Part model, mm, in its own coordinate system. Face numbers are marked on the shaded views. A direction names the side the tool comes from. Round coordinates to 2 decimals unless told otherwise and drop trailing zeros. Order: outer loops, then holes, each group sorted by start corner. A loop starts at its lowest first (then second) coordinate and runs counter-clockwise, first axis right, second up. Notation, with made-up numbers: (6, 9.5) - (32, 9.5) arc R12 cw to (32, 24.5) - close; hole circle Ø4 at (-13, 63.5). An arc over 180 degrees is marked (long way). Return JSON: item names as keys, results as strings. Group by question number.
Item 1: Saw through at A-A on y = -28. List the corners of the cut face in (x, z).
Item 2: Drop flat-ended pins along their axis: pin 1 (3 mm diameter, centred on y = -13, z = 0.5, fed in from -X); pin 2 (5 mm diameter, centred on y = 3.5, z = 3, fed in from +X); pin 3 (3 mm diameter, centred on y = -27.5, z = 2, fed in from +X). Give the stop position or say it passes through.
Item 3: Probe probe 1 along X at (y, z) = (26.25, 0); probe 2 along Z at (x, y) = (-25, 23.5); probe 3 along Y at (x, z) = (-17, -4.5). List the from-to ranges inside material, lowest first.
Item 4: Saw through at D-D on z = 3.5. List the corners of the cut face in (x, y).
Item 5: Two-plate mould, pull along Y, no slides. Class the marked faces 1, 2, 3 and 4: released by +Y, released by -Y, zero draft, split by the parting line, or undercut.
Item 6: Tool access for the marked faces 5 and 6: list every direction of +Z, -Z, +X, -X, +Y, -Y with a clear straight run to the whole face (end or side of a thin tool).
Item 7: Saw through at C-C on y = -13.5. List the corners of the cut face in (x, z).
Item 8: Saw through at B-B on z = 0. State how many separate pieces and enclosed holes the cut face has, and give its area (3 significant figures).
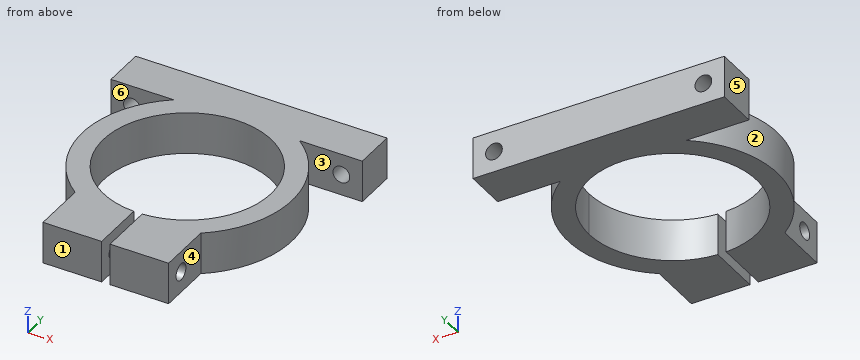
```python
from build123d import *

# Parameters (mm, degrees)
CYLINDER002_R     = 2
CYLINDER002_DEPTH = 10
CYLINDER001_R     = 20
CYLINDER001_DEPTH = 10
CYLINDER004_R     = 2
CYLINDER004_DEPTH = 30
BOX002_W          = 2
BOX002_H          = 15
BOX002_DEPTH      = 10
CYLINDER003_R     = 2
CYLINDER003_DEPTH = 10
BOX_W             = 60
BOX_H             = 10
BOX_DEPTH         = 10
BOX001_W          = 30
BOX001_H          = 15
BOX001_DEPTH      = 10
CYLINDER_R        = 25
CYLINDER_DEPTH    = 10


with BuildPart() as cylinder002:
    # Cylinder002 → Cylinder002 (new body)
    with BuildSketch(Plane(origin=(25, 20, 0), x_dir=(1, 0, 0), z_dir=(0, 1, 0))):
        Circle(CYLINDER002_R)
    extrude(amount=CYLINDER002_DEPTH)


with BuildPart() as cylinder001:
    # Cylinder001 → Cylinder001 (new body)
    with BuildSketch(Plane.XY.offset(-5)):
        Circle(CYLINDER001_R)
    extrude(amount=CYLINDER001_DEPTH)


with BuildPart() as cylinder004:
    # Cylinder004 → Cylinder004 (new body)
    with BuildSketch(Plane(origin=(-15, -28, 0), x_dir=(0, 0, -1), z_dir=(1, 0, 0))):
        Circle(CYLINDER004_R)
    extrude(amount=CYLINDER004_DEPTH)


with BuildPart() as cube002:
    # Box002 → Box002 (new body)
    with BuildSketch(Plane(origin=(-1, -33, -5), x_dir=(1, 0, 0), z_dir=(0, 0, 1))):
        with Locations((1, 7.5)):
            Rectangle(BOX002_W, BOX002_H)
    extrude(amount=BOX002_DEPTH)


with BuildPart() as negative_fusion:
    # Cylinder003 → Cylinder003 (new body)
    with BuildSketch(Plane(origin=(-25, 20, 0), x_dir=(1, 0, 0), z_dir=(0, 1, 0))):
        Circle(CYLINDER003_R)
    extrude(amount=CYLINDER003_DEPTH)

    # Fusion001: union Cylinder002, Cylinder001, Cylinder004, Cube002
    add(cylinder002.part)
    add(cylinder001.part)
    add(cylinder004.part)
    add(cube002.part)


with BuildPart() as cube:
    # Box → Box (new body)
    with BuildSketch(Plane(origin=(-30, 20, -5), x_dir=(1, 0, 0), z_dir=(0, 0, 1))):
        with Locations((30, 5)):
            Rectangle(BOX_W, BOX_H)
    extrude(amount=BOX_DEPTH)


with BuildPart() as cube001:
    # Box001 → Box001 (new body)
    with BuildSketch(Plane(origin=(-15, -33, -5), x_dir=(1, 0, 0), z_dir=(0, 0, 1))):
        with Locations((15, 7.5)):
            Rectangle(BOX001_W, BOX001_H)
    extrude(amount=BOX001_DEPTH)


with BuildPart() as cut:
    # Cylinder → Cylinder (new body)
    with BuildSketch(Plane.XY.offset(-5)):
        Circle(CYLINDER_R)
    extrude(amount=CYLINDER_DEPTH)

    # Fusion: union Cube, Cube001
    add(cube.part)
    add(cube001.part)

    # Cut: cut Negative Fusion
    add(negative_fusion.part, mode=Mode.SUBTRACT)


solid = cut.part
```
Filled in:
{
 "1": {"outline": "(-15, -5) - (-1, -5) - (-1, -2) - (-15, -2) - close; (-15, 2) - (-1, 2) - (-1, 5) - (-15, 5) - close; (1, -5) - (15, -5) - (15, -2) - (1, -2) - close; (1, 2) - (15, 2) - (15, 5) - (1, 5) - close"},
 "2": {"pin 1": "stops at x = -22.2", "pin 2": "stops at x = 24.98", "pin 3": "stops at x = 15"},
 "3": {"probe 1": "x = -30 to -27, -23 to 23, 27 to 30", "probe 2": "z = -5 to -2, 2 to 5", "probe 3": "y = -18.33 to -10.54, 10.54 to 18.33, 20 to 30"},
 "4": {"outline": "(-30, 20) - (-15, 20) arc R25 ccw to (-15, -20) - (-15, -33) - (-1, -33) - (-1, -19.97) arc R20 cw (long way) to (1, -19.97) - (1, -33) - (15, -33) - (15, -20) arc R25 ccw to (15, 20) - (30, 20) - (30, 30) - (-30, 30) - close"},
 "5": {"face 1": "released by -Y", "face 2": "undercut", "face 3": "undercut", "face 4": "zero draft"},
 "6": {"face 5": "+Z, -Z, -X, +Y, -Y", "face 6": "+Z, -Z, -X"},
 "7": {"outline": "(-21.04, -5) - (-14.76, -5) - (-14.76, 5) - (-21.04, 5) - close; (14.76, -5) - (21.04, -5) - (21.04, 5) - (14.76, 5) - close"},
 "8": {"separate pieces": "5", "enclosed holes": "0", "area": "1,270 mm^2"}
}
